Here's how the part is built. I have some questions about the finished solid (model axes, mm). A direction names the side the tool comes from. Coordinates: 2 decimals unless noted, no trailing zeros. Write each loop counter-clockwise with the first axis right and the second up, starting at its lowest first coordinate (ties: lowest second). Pieces come first, ordered by that corner, then holes.
Item 1: I want a section at A-A (y = 15). Count the separate pieces of the cut face and the enclosed holes in it, and give its area (3 significant figures).
Item 2: For faces 1 (the face through (5.494, 15.394, 25.257)), 2 (the face through (-23, 12.859, -10)), 3 (the face through (-18.75, 15.39, -9.73)), which set-ups out of +Z, -Z, +X, -X, +Y, -Y let a thin tool reach every point of the face, with its end or its side?
Item 3: I want a section at B-B (x = 65.5). Please give me the cut outline in (y, z).
Item 4: Please list where these lines run through material, in increasing order: line 1 (Z direction, x = -4, y = 19.5); line 2 (Z direction, x = 4.5, y = 19.25); line 3 (Y direction, x = 12.5, z = -25).
Item 5: If we mould it in two halves opening along X, with no side actions, what happens to faces 4 (the face through (-45.636, 19.38, 59.517)), 5 (the face through (2, 17.859, -22)), 6 (the face through (2.99, 15.394, -31.237)), 7 (the face through (-18, 12.859, 20))? For each: pulls with the +X half, pulls with the -X half, needs draft (parallel to the pull), parting line crosses it, or undercut.
Item 6: I want a section at C-C (z = 53.5). Please give me the cut outline in (x, y), and give its area (3 significant figures).
Item 7: I'm going to push flat-ended pins straight in: P1, Ø3, axis at x = -4.89, z = 1.06, coming from the -Y side; P2, Ø3, axis at x = 45, y = 14.5, coming from the -Z side; P3, Ø1.5, axis at y = 19, z = -12, coming from the -X side; P4, Ø1.5, axis at x = 5.5, y = 16.5, coming from the -Z side. Where does each tip first touch, or does it pass through?
from build123d import *

# Parameters (mm, degrees)
SKETCH_2_R               = 75
EXTRUDE_1_DEPTH          = 3
SKETCH_3_R               = 1.599999866
EXTRUDE_2_DEPTH          = 5
CUT_EXTRUDE_1_DEPTH      = 10
CUT_EXTRUDE_1_DEPTH_BACK = 107.367288205
SKETCH_18_R              = 1.5
SKETCH_18_R_2            = 1
SKETCH_18_R_3            = 1.6


with BuildPart() as part:
    # 草图1 → 旋转1 (revolve)
    with BuildSketch(Plane.XY, mode=Mode.PRIVATE) as revolve_1_sk:
        Polygon((0, 20.860199313), (-13.879633592, 20.860199313), (-17.5, 20.860199313), (-17.5, 20.859199313), (0, 20.859199313), align=None)
    revolve(revolve_1_sk.sketch.rotate(Axis((0, 0, 0), (0, 1, 0)), 270), axis=Axis((0, 0, 0), (0, 1, 0)))

    # 草图2 → 凸台-拉伸1 (add)
    with BuildSketch(Plane.XZ.offset(-20.859199313)):
        with Locations(Location((0, 0, 0), (0, 0, 270))):
            Circle(SKETCH_2_R)
    extrude(amount=EXTRUDE_1_DEPTH)

    # 草图3 → 凸台-拉伸2 (add)
    # profile 1 of 6: a face of its own
    with BuildSketch(Plane(origin=(0, 17.859199313, 0), x_dir=(-1, 0, 0), z_dir=(0, -1, 0))):
        with BuildLine():
            Line((-2.033163228, 20.270074719), (-1.846291915, 18.407019447))
            ThreePointArc((-1.846291915, 18.407019447), (1.055931242, 18.469222181), (3.932153868, 18.076651369))
            Line((3.932153868, 18.076651369), (7.013047727, 32.239943565))
            Line((7.013047727, 32.239943565), (-3.131720421, 31.222385917))
            Line((-3.131720421, 31.222385917), (-2.352464069, 23.453415742))
            ThreePointArc((-2.352464069, 23.453415742), (-1.140108901, 23.033755173), (-0.625758844, 21.858440719))
            ThreePointArc((-0.625758844, 21.858440719), (-1.028229521, 20.797345336), (-2.033163228, 20.270074719))
        make_face()
    # profile 2 of 6: a face of its own
    with BuildSketch(Plane(origin=(0, 17.859199313, 0), x_dir=(-1, 0, 0), z_dir=(0, -1, 0))):
        with BuildLine():
            ThreePointArc((-7.444009782, 16.935580213), (-4.703053238, 17.891574805), (-1.846291915, 18.407019447))
            Line((-1.846291915, 18.407019447), (-2.033163228, 20.270074719))
            ThreePointArc((-2.033163228, 20.270074719), (-3.817770139, 21.698756103), (-2.352464069, 23.453415742))
            Line((-2.352464069, 23.453415742), (-3.131720421, 31.222385917))
            Line((-3.131720421, 31.222385917), (-13.276488569, 30.204828269))
            Line((-13.276488569, 30.204828269), (-7.444009782, 16.935580213))
        make_face()
    # profile 3 of 6: a face of its own
    with BuildSketch(Plane(origin=(0, 17.859199313, 0), x_dir=(-1, 0, 0), z_dir=(0, -1, 0))):
        with BuildLine():
            Line((24.623838156, 21.960496214), (13.80636839, 12.313056106))
            ThreePointArc((13.80636839, 12.313056106), (16.935580213, 7.444009782), (18.407019447, 1.846291915))
            Line((18.407019447, 1.846291915), (32.829159342, 3.292885719))
            Line((32.829159342, 3.292885719), (24.623838156, 21.960496214))
        make_face()
        with Locations(Location((20.100815215, 8.871451977, 0), (0, 0, 90))):
            Circle(SKETCH_3_R, mode=Mode.SUBTRACT)
    # profile 4 of 6: a face of its own
    with BuildSketch(Plane(origin=(0, 17.859199313, 0), x_dir=(-1, 0, 0), z_dir=(0, -1, 0))):
        with BuildLine():
            ThreePointArc((15.976814708, -9.325693034), (12.313056106, -13.80636839), (7.444009782, -16.935580213))
            Line((7.444009782, -16.935580213), (13.276488569, -30.204828269))
            Line((13.276488569, -30.204828269), (28.494857482, -16.632495199))
            Line((28.494857482, -16.632495199), (15.976814708, -9.325693034))
        make_face()
        with Locations(Location((14.648745714, -16.375581868, 0), (0, 0, 90))):
            Circle(SKETCH_3_R, mode=Mode.SUBTRACT)
    # profile 5 of 6: a face of its own
    with BuildSketch(Plane(origin=(0, 17.859199313, 0), x_dir=(-1, 0, 0), z_dir=(0, -1, 0))):
        with BuildLine():
            Line((-7.013047727, -32.239943565), (-3.932153868, -18.076651369))
            ThreePointArc((-3.932153868, -18.076651369), (-9.325693034, -15.976814708), (-13.80636839, -12.313056106))
            Line((-13.80636839, -12.313056106), (-24.623838156, -21.960496214))
            Line((-24.623838156, -21.960496214), (-7.013047727, -32.239943565))
        make_face()
        with Locations(Location((-11.047392472, -18.992118157, 0), (0, 0, 90))):
            Circle(SKETCH_3_R, mode=Mode.SUBTRACT)
    # profile 6 of 6: a face of its own
    with BuildSketch(Plane(origin=(0, 17.859199313, 0), x_dir=(-1, 0, 0), z_dir=(0, -1, 0))):
        with BuildLine():
            Line((-32.829159342, -3.292885719), (-18.407019447, -1.846291915))
            ThreePointArc((-18.407019447, -1.846291915), (-18.076651369, 3.932153868), (-15.976814708, 9.325693034))
            Line((-15.976814708, 9.325693034), (-28.494857482, 16.632495199))
            Line((-28.494857482, 16.632495199), (-32.829159342, -3.292885719))
        make_face()
        with Locations(Location((-21.476409748, 4.637807329, 0), (0, 0, 90))):
            Circle(SKETCH_3_R, mode=Mode.SUBTRACT)
    extrude(amount=EXTRUDE_2_DEPTH)

    # 草图18 → 切除-拉伸1 (cut, two sides: drawn at the far end of the back side and taken through both)
    with BuildSketch(Plane(origin=(0, 20.859199313, 0), x_dir=(1, 0, 0), z_dir=(0, 1, 0)).offset(-CUT_EXTRUDE_1_DEPTH_BACK)):
        with Locations(Location((1.98e-07, 1.15e-07, 0), (0, 0, 90))):
            Circle(SKETCH_18_R)
        with Locations(Location((2.94033472, 7.786611797, 0), (0, 0, 90))):
            Circle(SKETCH_18_R_2)
        with Locations(Location((4.940484912, 10.022545429, 0), (0, 0, 90))):
            Circle(SKETCH_18_R_2)
        with Locations(Location((7.176418545, 8.022395237, 0), (0, 0, 90))):
            Circle(SKETCH_18_R_2)
        with Locations(Location((9.412352177, 6.022245045, 0), (0, 0, 90))):
            Circle(SKETCH_18_R_2)
        with Locations(Location((7.412201985, 3.786311413, 0), (0, 0, 90))):
            Circle(SKETCH_18_R_2)
        with Locations(Location((3.333583851, 3.726556169, 0), (0, 0, 90))):
            Circle(SKETCH_18_R_2)
        with Locations(Location((-0.50651094, -4.974278372, 0), (0, 0, 90))):
            Circle(SKETCH_18_R_2)
        with Locations(Location((8.6360722, -7.090702541, 0), (0, 0, 90))):
            Circle(SKETCH_18_R_2)
        with Locations(Location((9.847386583, -4.34612289, 0), (0, 0, 90))):
            Circle(SKETCH_18_R_2)
        with Locations(Location((11.058700966, -1.601543238, 0), (0, 0, 90))):
            Circle(SKETCH_18_R_2)
        with Locations(Location((8.314121314, -0.390228855, 0), (0, 0, 90))):
            Circle(SKETCH_18_R_2)
        with Locations(Location((4.574299617, -2.01885719, 0), (0, 0, 90))):
            Circle(SKETCH_18_R_2)
        with Locations(Location((5.891492548, -5.879388159, 0), (0, 0, 90))):
            Circle(SKETCH_18_R_2)
        with Locations(Location((6.372601501, -10.955453391, 0), (0, 0, 90))):
            Circle(SKETCH_18_R_3)
        with Locations(Location((2.198075111, -8.027786333, 0), (0, 0, 90))):
            Circle(SKETCH_18_R_2)
        with Locations(Location((1.894168429, -11.012353426, 0), (0, 0, 90))):
            Circle(SKETCH_18_R_2)
        with Locations(Location((-1.090398663, -10.708446744, 0), (0, 0, 90))):
            Circle(SKETCH_18_R_2)
        with Locations(Location((-4.074965755, -10.404540061, 0), (0, 0, 90))):
            Circle(SKETCH_18_R_2)
        with Locations(Location((-8.450013147, -9.446125195, 0), (0, 0, 90))):
            Circle(SKETCH_18_R_3)
        with Locations(Location((-3.771059073, -7.419972969, 0), (0, 0, 90))):
            Circle(SKETCH_18_R_2)
        with Locations(Location((-9.888040223, -5.204465317, 0), (0, 0, 90))):
            Circle(SKETCH_18_R_2)
        with Locations(Location((-6.955635912, -4.571215795, 0), (0, 0, 90))):
            Circle(SKETCH_18_R_2)
        with Locations(Location((-4.887340321, -1.055415755, 0), (0, 0, 90))):
            Circle(SKETCH_18_R_2)
        with Locations(Location((-10.521289745, -2.272061006, 0), (0, 0, 90))):
            Circle(SKETCH_18_R_2)
        with Locations(Location((-11.154539267, 0.660343305, 0), (0, 0, 90))):
            Circle(SKETCH_18_R_2)
        with Locations(Location((-8.222134956, 1.293592827, 0), (0, 0, 90))):
            Circle(SKETCH_18_R_2)
        with Locations(Location((-2.51403122, 4.321995722, 0), (0, 0, 90))):
            Circle(SKETCH_18_R_2)
        with Locations(Location((-6.496894246, 5.202619761, 0), (0, 0, 90))):
            Circle(SKETCH_18_R_2)
        with Locations(Location((-1.310499517, 8.219457462, 0), (0, 0, 90))):
            Circle(SKETCH_18_R_2)
        with Locations(Location((-2.818918367, 10.812654827, 0), (0, 0, 90))):
            Circle(SKETCH_18_R_2)
        with Locations(Location((-5.412115732, 9.304235976, 0), (0, 0, 90))):
            Circle(SKETCH_18_R_2)
        with Locations(Location((-8.005313096, 7.795817125, 0), (0, 0, 90))):
            Circle(SKETCH_18_R_2)
        with Locations(Location((-11.594996558, 5.117427117, 0), (0, 0, 90))):
            Circle(SKETCH_18_R_3)
    extrude(amount=CUT_EXTRUDE_1_DEPTH + CUT_EXTRUDE_1_DEPTH_BACK, mode=Mode.SUBTRACT)


solid = part.part
Answer:
1. separate pieces: 5
1. enclosed holes: 5
1. area: 1,020 mm2
2. face 1: +Z, -Y
2. face 2: +Z, -Z, +X, -X, -Y
2. face 3: -Y
3. outline: (17.86, -36.53) - (20.86, -36.53) - (20.86, 36.53) - (17.86, 36.53) - close
4. line 1: z = -74.89 to 0.59, 1.52 to 6.45, 8.39 to 9.41, 11.4 to 74.89
4. line 2: z = -74.86 to -10.92, -9.12 to 1.02, 3.02 to 74.86
4. line 3: y = 17.86 to 20.86
5. face 4: parting line crosses it
5. face 5: undercut
5. face 6: pulls with the +X half
5. face 7: needs draft
6. outline: (-52.56, 17.86) - (52.56, 17.86) - (52.56, 20.86) - (-52.56, 20.86) - close
6. area: 315 mm2
7. P1: stops at y = 17.86
7. P2: passes through
7. P3: stops at x = -74.15
7. P4: stops at z = -31.06
